```python
from build123d import *

# Parameters (mm, degrees)
SM_BASE_FLANGE_1_DEPTH = 70
CUT_EXTRUDE_7_REACH    = 79.105
SKETCH_18_W            = 40.5
SKETCH_18_H            = 20.5
CUT_EXTRUDE_8_REACH    = 79.105
SKETCH_19_R            = 2.1
FILLET_2_R             = 1
CUT_EXTRUDE_9_REACH    = 81.783
SKETCH_20_R            = 2.1
CHAMFER_3_SIZE         = 5


# Sheet-metal steps are written as plain solids
with BuildPart() as part:
    # Sketch 1 → 基材-凸緣1 (new body)
    with BuildSketch(Plane.XY):
        with BuildLine():
            Line((-12.5, 17.5), (-12.5, -16))
            ThreePointArc((-12.5, -16), (-12.060660172, -17.060660172), (-11, -17.5))
            Line((-11, -17.5), (12.5, -17.5))
            Line((12.5, -17.5), (12.5, -20.5))
            Line((12.5, -20.5), (-11, -20.5))
            ThreePointArc((-11, -20.5), (-14.181980515, -19.181980515), (-15.5, -16))
            Line((-15.5, -16), (-15.5, 17.5))
            Line((-15.5, 17.5), (-12.5, 17.5))
        make_face()
    extrude(amount=SM_BASE_FLANGE_1_DEPTH)

    # 草圖18 → 除料-伸長7 (cut, up to next)
    with BuildSketch(Plane(origin=(-12.5, 0, 0), x_dir=(0, 0, -1), z_dir=(1, 0, 0)), mode=Mode.PRIVATE) as cut_extrude_7_sk1:
        with Locations((-35, 0.75)):
            Rectangle(SKETCH_18_W, SKETCH_18_H)
    cut_extrude_7_tool1 = extrude(cut_extrude_7_sk1.sketch, amount=-CUT_EXTRUDE_7_REACH, mode=Mode.PRIVATE) & part.part
    add(cut_extrude_7_tool1.solids().sort_by_distance((-12.5, 0.75, 35))[0], mode=Mode.SUBTRACT)

    # 草圖19 → 除料-伸長8 (cut, up to next)
    with BuildSketch(Plane(origin=(-12.5, 0, 0), x_dir=(0, 0, -1), z_dir=(1, 0, 0)), mode=Mode.PRIVATE) as cut_extrude_8_sk1:
        with Locations(Location((-10.25, 5.75, 0), (0, 0, 90))):
            Circle(SKETCH_19_R)
    cut_extrude_8_tool1 = extrude(cut_extrude_8_sk1.sketch, amount=-CUT_EXTRUDE_8_REACH, mode=Mode.PRIVATE) & part.part
    # 草圖19 → 除料-伸長8 (cut, up to next)
    with BuildSketch(Plane(origin=(-12.5, 0, 0), x_dir=(0, 0, -1), z_dir=(1, 0, 0)), mode=Mode.PRIVATE) as cut_extrude_8_sk2:
        with Locations(Location((-10.25, -4.25, 0), (0, 0, 90))):
            Circle(SKETCH_19_R)
    cut_extrude_8_tool2 = extrude(cut_extrude_8_sk2.sketch, amount=-CUT_EXTRUDE_8_REACH, mode=Mode.PRIVATE) & part.part
    # 草圖19 → 除料-伸長8 (cut, up to next)
    with BuildSketch(Plane(origin=(-12.5, 0, 0), x_dir=(0, 0, -1), z_dir=(1, 0, 0)), mode=Mode.PRIVATE) as cut_extrude_8_sk3:
        with Locations(Location((-59.75, -4.25, 0), (0, 0, 90))):
            Circle(SKETCH_19_R)
    cut_extrude_8_tool3 = extrude(cut_extrude_8_sk3.sketch, amount=-CUT_EXTRUDE_8_REACH, mode=Mode.PRIVATE) & part.part
    # 草圖19 → 除料-伸長8 (cut, up to next)
    with BuildSketch(Plane(origin=(-12.5, 0, 0), x_dir=(0, 0, -1), z_dir=(1, 0, 0)), mode=Mode.PRIVATE) as cut_extrude_8_sk4:
        with Locations(Location((-59.75, 5.75, 0), (0, 0, 90))):
            Circle(SKETCH_19_R)
    cut_extrude_8_tool4 = extrude(cut_extrude_8_sk4.sketch, amount=-CUT_EXTRUDE_8_REACH, mode=Mode.PRIVATE) & part.part
    add(cut_extrude_8_tool1.solids().sort_by_distance((-12.5, 5.75, 10.25))[0], mode=Mode.SUBTRACT)
    add(cut_extrude_8_tool2.solids().sort_by_distance((-12.5, -4.25, 10.25))[0], mode=Mode.SUBTRACT)
    add(cut_extrude_8_tool3.solids().sort_by_distance((-12.5, -4.25, 59.75))[0], mode=Mode.SUBTRACT)
    add(cut_extrude_8_tool4.solids().sort_by_distance((-12.5, 5.75, 59.75))[0], mode=Mode.SUBTRACT)

    # 圓角2
    fillet_2_edges = [part.edges().sort_by_distance(p)[0] for p in [
        (-14, 11, 14.75),
        (-14, -9.5, 14.75),
        (-14, -9.5, 55.25),
        (-14, 11, 55.25),
    ]]
    fillet(fillet_2_edges, radius=FILLET_2_R)

    # 草圖20 → 除料-伸長9 (cut, up to next)
    with BuildSketch(Plane(origin=(0, -17.5, 0), x_dir=(1, 0, 0), z_dir=(0, 1, 0)), mode=Mode.PRIVATE) as cut_extrude_9_sk1:
        with Locations(Location((-5.5, -15, 0), (0, 0, 270))):
            Circle(SKETCH_20_R)
    cut_extrude_9_tool1 = extrude(cut_extrude_9_sk1.sketch, amount=-CUT_EXTRUDE_9_REACH, mode=Mode.PRIVATE) & part.part
    # 草圖20 → 除料-伸長9 (cut, up to next)
    with BuildSketch(Plane(origin=(0, -17.5, 0), x_dir=(1, 0, 0), z_dir=(0, 1, 0)), mode=Mode.PRIVATE) as cut_extrude_9_sk2:
        with Locations(Location((7, -15, 0), (0, 0, 270))):
            Circle(SKETCH_20_R)
    cut_extrude_9_tool2 = extrude(cut_extrude_9_sk2.sketch, amount=-CUT_EXTRUDE_9_REACH, mode=Mode.PRIVATE) & part.part
    # 草圖20 → 除料-伸長9 (cut, up to next)
    with BuildSketch(Plane(origin=(0, -17.5, 0), x_dir=(1, 0, 0), z_dir=(0, 1, 0)), mode=Mode.PRIVATE) as cut_extrude_9_sk3:
        with Locations(Location((7, -55, 0), (0, 0, 270))):
            Circle(SKETCH_20_R)
    cut_extrude_9_tool3 = extrude(cut_extrude_9_sk3.sketch, amount=-CUT_EXTRUDE_9_REACH, mode=Mode.PRIVATE) & part.part
    # 草圖20 → 除料-伸長9 (cut, up to next)
    with BuildSketch(Plane(origin=(0, -17.5, 0), x_dir=(1, 0, 0), z_dir=(0, 1, 0)), mode=Mode.PRIVATE) as cut_extrude_9_sk4:
        with Locations(Location((-5.5, -55, 0), (0, 0, 270))):
            Circle(SKETCH_20_R)
    cut_extrude_9_tool4 = extrude(cut_extrude_9_sk4.sketch, amount=-CUT_EXTRUDE_9_REACH, mode=Mode.PRIVATE) & part.part
    add(cut_extrude_9_tool1.solids().sort_by_distance((-5.5, -17.5, 15))[0], mode=Mode.SUBTRACT)
    add(cut_extrude_9_tool2.solids().sort_by_distance((7, -17.5, 15))[0], mode=Mode.SUBTRACT)
    add(cut_extrude_9_tool3.solids().sort_by_distance((7, -17.5, 55))[0], mode=Mode.SUBTRACT)
    add(cut_extrude_9_tool4.solids().sort_by_distance((-5.5, -17.5, 55))[0], mode=Mode.SUBTRACT)

    # 導角3
    chamfer_3_edges = [part.edges().sort_by_distance(p)[0] for p in [
        (-14, 17.5, 70),
        (-14, 17.5, 0),
        (12.5, -19, 70),
        (12.5, -19, 0),
    ]]
    chamfer(chamfer_3_edges, length=CHAMFER_3_SIZE)


solid = part.part
```
The listing builds one solid part. Answer for the finished solid, in the listing's coordinates (mm). A direction names the side the tool comes from. Round coordinates to 2 decimals unless told otherwise and drop trailing zeros. Loops run counter-clockwise (first coordinate to the right, second up) from the corner with the lowest first, then second, coordinate; pieces in that order, holes last. Notation, with made-up numbers: (58.5, -6.5) - (78.5, -6.5) arc R31 ccw to (78.5, 17.5) - close; hole circle Ø5 at (20, -12). An arc over 180 degrees is marked (long way). Use one line per item in the form item = value. Start each with the question number.
1. For a pull along X with two mould halves and no side action, classify faces 4 (the face through (-6.3, -18.98, 56.94)), 5 (the face through (-13, -9, 0)), 6 (the face through (10, -19, 2.5)) as pulls with the +X half, pulls with the -X half, needs draft (parallel to the pull), parting line crosses it, or undercut.
2. The part is cut by section C-C on z = 48. Determine the outline of the cut face in (x, y).
3. A tool of negligible diameter and unlimited length cuts with its end or side. For faces 1 (the face through (-14, 1, 55.25)), 2 (the face through (1, -20.5, 35)), 3 (the face through (1, -17.5, 35)), from which of +Z, -Z, +X, -X, +Y, -Y can it reach the whole face along a straight path? Write none if from no direction.
4. The part is cut by section B-B on z = 10.25. Determine the outline of the cut face in (x, y).
5. Consider line 1 (Z direction, x = -13.5, y = -4.25); line 2 (X direction, y = -19, z = 55); line 3 (X direction, y = -18.35, z = 15). Determine where each line is inside the solid, lowest interval first. Write a range as [from, to].
6. The part is cut by section A-A on x = -5.5. Determine the outline of the cut face in (y, z), then the cut area to 3 significant figures.
7. The part is cut by section D-D on y = -3. Determine the outline of the cut face in (x, z).
8. Given pin 1 Ø3 at (y, z) = (2.5, 54.5) entering from +X; pin 2 Ø12 at (x, z) = (-0.5, 38) entering from +Y; pin 3 Ø1.5 at (x, z) = (-13.5, 31) entering from -Y, each flat-ended and moving along its own axis, determine where each tip first touches the part or whether it passes through.
Geometry check:
q1.face_4 = undercut
q1.face_5 = needs draft
q1.face_6 = pulls with the +X half
q2.outline = (-15.5, -16) arc R4.5 ccw to (-11, -20.5) - (12.5, -20.5) - (12.5, -17.5) - (-11, -17.5) arc R1.5 cw to (-12.5, -16) - (-12.5, -9.5) - (-15.5, -9.5) - close; (-15.5, 11) - (-12.5, 11) - (-12.5, 17.5) - (-15.5, 17.5) - close
q3.face_1 = +X, -X
q3.face_2 = +Z, -Z, +X, -X, -Y
q3.face_3 = +Z, -Z, +X, +Y
q4.outline = (-15.5, -16) arc R4.5 ccw to (-11, -20.5) - (12.5, -20.5) - (12.5, -17.5) - (-11, -17.5) arc R1.5 cw to (-12.5, -16) - (-12.5, -6.35) - (-15.5, -6.35) - close; (-15.5, -2.15) - (-12.5, -2.15) - (-12.5, 3.65) - (-15.5, 3.65) - close; (-15.5, 7.85) - (-12.5, 7.85) - (-12.5, 17.5) - (-15.5, 17.5) - close
q5.line_1 = [0, 8.15], [12.35, 14.75], [55.25, 57.65], [61.85, 70]
q5.line_2 = [-14.35, -7.6], [-3.4, 4.9], [9.1, 12.5]
q5.line_3 = [-14.84, -7.6], [-3.4, 4.9], [9.1, 12.5]
q6.outline = (-20.5, 0) - (-17.5, 0) - (-17.5, 12.9) - (-20.5, 12.9) - close; (-20.5, 17.1) - (-17.5, 17.1) - (-17.5, 52.9) - (-20.5, 52.9) - close; (-20.5, 57.1) - (-17.5, 57.1) - (-17.5, 70) - (-20.5, 70) - close
q6.area = 185 mm^2
q7.outline = (-15.5, 0) - (-12.5, 0) - (-12.5, 8.56) - (-15.5, 8.56) - close; (-15.5, 11.94) - (-12.5, 11.94) - (-12.5, 14.75) - (-15.5, 14.75) - close; (-15.5, 55.25) - (-12.5, 55.25) - (-12.5, 58.06) - (-15.5, 58.06) - close; (-15.5, 61.44) - (-12.5, 61.44) - (-12.5, 70) - (-15.5, 70) - close
q8.pin_1 = -12.5
q8.pin_2 = -17.5
q8.pin_3 = -20.15
